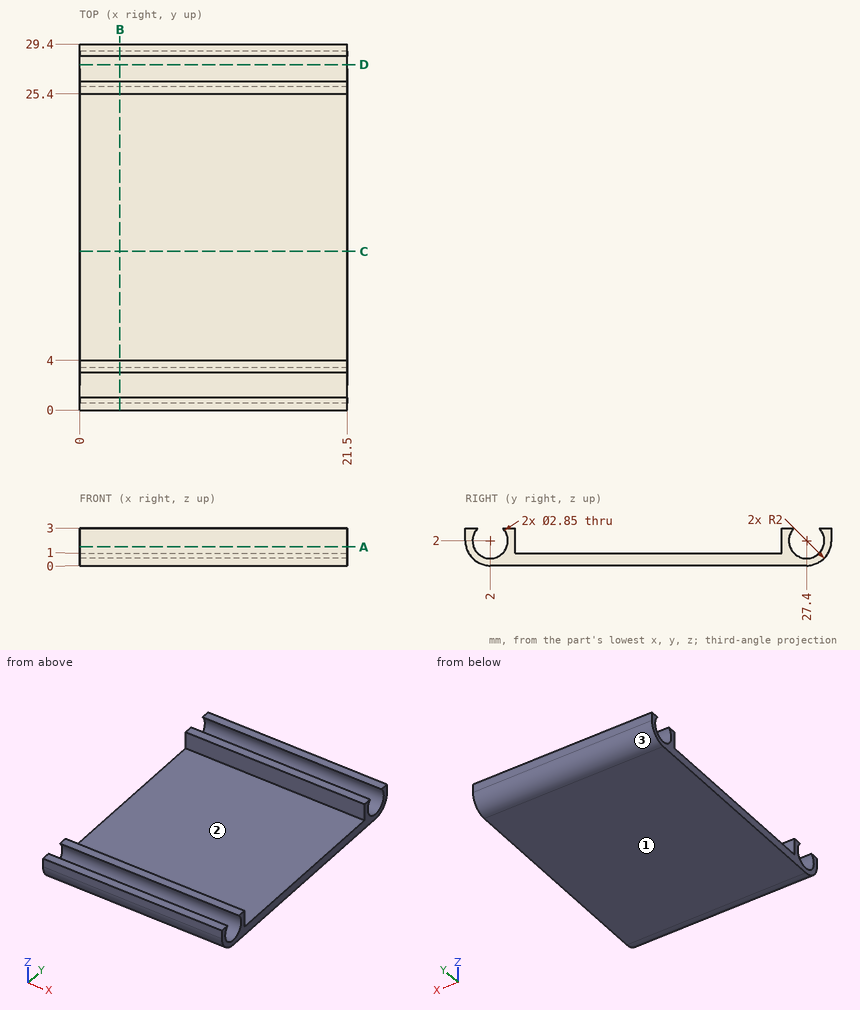
Answer from the drawing. Dimensions are ordinates in mm from the lowest x, y and z of the part. Round coordinates to 2 decimals unless told otherwise and drop trailing zeros. Order: outer loops, then holes, each group sorted by start corner. A loop starts at its lowest first (then second) coordinate and runs counter-clockwise, first axis right, second up. Notation, with made-up numbers: (-0.5, 1.5) -> (11.5, 1.5) arc R26 cw to (11.5, 19.5) -> close; hole circle Ø2 at (47.25, 53.5). An arc over 180 degrees is marked (long way). Answer as CSV lines item,"result".
Q1. A cutting plane is placed at C-C on y = 12.75. Determine the outline of the cut face in (x, z), plus the area to 3 significant figures.
Computed values:
outline,"(0, 0) -> (21.5, 0) -> (21.5, 1) -> (0, 1) -> close"
area,"21.5 mm^2"
Q2. A cutting plane is placed at D-D on y = 27.75. Determine the outline of the cut face in (x, z).
Computed values:
outline,"(0, 0.03) -> (21.5, 0.03) -> (21.5, 0.62) -> (0, 0.62) -> close"
Q3. A cutting plane is placed at A-A on z = 1.5. Determine the outline of the cut face in (x, y).
Computed values:
outline,"(0, 0.06) -> (21.5, 0.06) -> (21.5, 0.67) -> (0, 0.67) -> close; (0, 3.33) -> (21.5, 3.33) -> (21.5, 4) -> (0, 4) -> close; (0, 25.4) -> (21.5, 25.4) -> (21.5, 26.07) -> (0, 26.07) -> close; (0, 28.73) -> (21.5, 28.73) -> (21.5, 29.34) -> (0, 29.34) -> close"
Q4. Given pin 1 (1 mm diameter, centred on x = 18, y = 6.5, fed in from +Z), flat-ended and moving along its own axis, determine where the tip first touches the part or whether it passes through.
Computed values:
pin 1,"stops at z = 1"
Q5. For a pull along Y with two mould halves and no side action, classify the marked faces 1, 2 and 3 as +Y half, -Y half, draft (parallel to the pull), parting line (faces both ways), or undercut.
Computed values:
face 1,"draft"
face 2,"undercut"
face 3,"+Y half"
Q6. A cutting plane is placed at B-B on x = 3.25. Determine the outline of the cut face in (y, z) (3 decimals).
Computed values:
outline,"(0, 2) arc R2 ccw to (2, 0) -> (27.4, 0) arc R2 ccw to (29.4, 2) -> (29.4, 3) -> (28.415, 3) arc R1.425 cw (long way) to (26.385, 3) -> (25.4, 3) -> (25.4, 1) -> (4, 1) -> (4, 3) -> (3.015, 3) arc R1.425 cw (long way) to (0.985, 3) -> (0, 3) -> close"
Q7. Consider line 1 (Y direction, x = 16, z = 2) (3 decimals); line 2 (Y direction, x = 6, z = 2.8); line 3 (Y direction, x = 17, z = 0.8). Determine where each line is inside the solid, lowest interval first. Write a range as from..to.
Computed values:
line 1,"y = 0..0.575, 3.425..4, 25.4..25.975, 28.825..29.4"
line 2,"y = 0..0.82, 3.18..4, 25.4..26.22, 28.58..29.4"
line 3,"y = 0.4..1.23, 2.77..26.63, 28.17..29"
